Geometry: final body of the model. Coordinates: model frame, mm. Face numbers are marked on the shaded views. A direction names the side the tool comes from. Give positions to 0.01 mm unless a question says otherwise; leave off trailing zeros. Loops run counter-clockwise (first coordinate to the right, second up) from the corner with the lowest first, then second, coordinate; pieces in that order, holes last. Notation, with made-up numbers: (6, 4.5) - (22, 4.5) arc R22 cw to (22, 11.5) - close; hole circle Ø3 at (13.25, 81.25). An arc over 180 degrees is marked (long way). Use one line per item in the form item = value.
Autodesk Inventor part; units mm, degrees
ref_plane "YZ Plane" through (0, 0, 0) normal (1, 0, 0) x (0, 1, 0)
ref_plane "XZ Plane" through (0, 0, 0) normal (0, 1, 0) x (-1, 0, 0)
ref_plane "XY Plane" through (0, 0, 0) normal (0, 0, 1) x (1, 0, 0)
sketch "Sketch1" plane through (0, 0, 0) normal (0, 0, 1) x (1, 0, 0)
  circle A0 centre (-57, 57.5) radius 3
  circle A1 centre (57, 57.5) radius 3
  circle A2 centre (-57, -57.5) radius 3
  circle A3 centre (57, -57.5) radius 3
  line L0 (-57, -57.5) -> (57, 57.5) construction
  line L1 (-67.5, 67.5) -> (67.5, 67.5) construction
  line L2 (67.5, 67.5) -> (67.5, -67.5) construction
  line L3 (67.5, -67.5) -> (-67.5, -67.5) construction
  line L4 (-67.5, -67.5) -> (-67.5, 67.5) construction
  line L5 (-67.5, 67.5) -> (67.5, -67.5) construction
  line L6 (67.5, 67.5) -> (-67.5, -67.5) construction
  circle A4 centre (-37.5, 37.5) radius 4
  circle A5 centre (-37.5, -37.5) radius 4
  circle A6 centre (37.5, -37.5) radius 4
  circle A7 centre (37.5, 37.5) radius 4
  arc A8 (-48.5, 62.5) -> (-48.5, -62.5) centre (326.325, 0) ccw
  line L7 (0, 67.5) -> (0, -67.5) construction
  line L8 (67.5, -67.5) -> (67.5, 67.5) construction
  arc A9 (48.5, -62.5) -> (48.5, 62.5) centre (-326.325, 0) ccw
  arc A10 (48.5, 62.5) -> (-48.5, 62.5) centre (0, -110.8429) ccw
  line L9 (-67.5, 0) -> (53.675, 0) construction
  arc A11 (-48.5, -62.5) -> (48.5, -62.5) centre (0, 110.8429) ccw
  arc A12 (-30.7003, 46.1842) -> (-30.7003, -46.1842) centre (326.325, 0) ccw
  arc A13 (-30.7003, -46.1842) -> (30.7003, -46.1842) centre (0, 110.8429) ccw
  arc A14 (30.7003, -46.1842) -> (30.7003, 46.1842) centre (-326.325, 0) ccw
  arc A15 (30.7003, 46.1842) -> (-30.7003, 46.1842) centre (0, -110.8429) ccw
  point P0 (0, 0)
  point P1 (0, 0)
  point P2 (-53.675, 0)
  point P3 (0, 0)
  dimension "d0" = 114
  dimension "d1" = 115
  dimension "d2" = 6
  dimension "d3" = 135
  dimension "d4" = 135
  dimension "d5" = 8
  dimension "d9" = 360
  dimension "d29" = 75
  dimension "d30" = 125
  dimension "d31" = 97
  dimension "d32" = 180
  dimension "d33" = 380
  dimension "d34" = 20
extrude "Extrusion1" add sketch "Sketch1" along normal mid plane 220 contours A10 A9 A11 A8
fillet "Fillet2" radius 15 8 edges at (48.5, 62.5, 0) (-48.5, 62.5, 0) (-48.5, -62.5, 0) (48.5, -62.5, 0) (-30.7003, 46.1842, 0) (30.7003, 46.1842, 0) (30.7003, -46.1842, 0) (-30.7003, -46.1842, 0)
properties part number "lineaire as deel 1" material "Aluminum 6061"
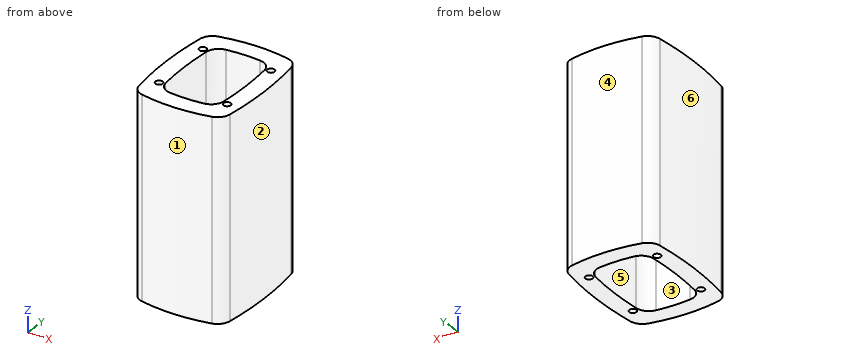
(1) Cut plane B-B (x = -13.5). Return the cut outline in (y, z).
Solution:
outline = (-68.65, -110) - (-48.59, -110) - (-48.59, 110) - (-68.65, 110) - close; (48.59, -110) - (68.65, -110) - (68.65, 110) - (48.59, 110) - close
(2) Cut plane C-C (z = -44). Give the number of separate pieces and of enclosed holes in the cut face, plus the area to 3 significant figures.
Solution:
separate_pieces = 1
enclosed_holes = 5
area = 7,400 mm2
(3) Pull-direction query (Y, two-part tool) for the marked faces 1, 2, 3 and 4; classes: released by +Y, released by -Y, zero draft, split by the parting line, or undercut.
Solution:
face_1 = released by -Y
face_2 = split by the parting line
face_3 = undercut
face_4 = released by +Y
(4) Access query for the marked faces 5 and 6. Directions: +Z, -Z, +X, -X, +Y, -Y. A direction counts if a zero-diameter tool reaches every point of the face in a straight line with its end or side. Return the directions, or none.
Solution:
face_5 = +Z, -Z
face_6 = +Z, -Z, -X
(5) Material intervals for L1, parallel to X at y = -0.5, z = 97; L2, parallel to Y at x = -37, z = -34; L3, parallel to Y at x = 35.5, z = 91.5, sorted ascending. Write a range as from..to.
Solution:
L1 = -53.67..-33.67, 33.67..53.67
L2 = -65.31..-41.47, -33.53..33.53, 41.47..65.31
L3 = -65.62..-40.96, -34.04..34.04, 40.96..65.62
(6) Cut plane A-A (y = 16). Return the cut outline in (x, z), plus the area to 3 significant figures.
Solution:
outline = (-53.34, -110) - (-33.32, -110) - (-33.32, 110) - (-53.34, 110) - close; (33.32, -110) - (53.34, -110) - (53.34, 110) - (33.32, 110) - close
area = 8,810 mm2
(7) Pin query (flat end, axial travel): P1, Ø1.5, axis at x = 36, z = -26, coming from the -Y side; P2, Ø1.5, axis at x = 42, z = -28.5, coming from the +Y side; P3, Ø4, axis at x = -19, z = 67.5, coming from the -Y side. Return the tip coordinate at first contact, or that it passes through.
Solution:
P1 = -65.67
P2 = 64.08
P3 = -68.35
